Read the model definition and answer for the solid it produces. Units are mm, in the model's axes. A direction names the side the tool comes from. Give positions to 0.01 mm unless a question says otherwise; leave off trailing zeros. Write each loop counter-clockwise with the first axis right and the second up, starting at its lowest first coordinate (ties: lowest second). Pieces come first, ordered by that corner, then holes. Notation, with made-up numbers: M 86.25,74 L 90.25,74 A22 cw 90.25,110 Z; hole C 40,-22 d10. An arc over 180 degrees is marked long. Answer as CSV lines item,"result". Start each with the question number.
```python
from build123d import *

# Parameters (mm, degrees)
SKETCH2_W          = 20.32
SKETCH2_H          = 20.32
CENTRAL_BOX_DEPTH  = 25.4
NIBBLES_DEPTH      = 6.35
NIBBLES_DEPTH_BACK = 31.75
SKETCH4_R          = 3.175
YAY_ROUNDED_R      = 2.54


with BuildPart() as part:
    # Sketch2 → central box (new body)
    with BuildSketch(Plane(origin=(0, 0, 0), x_dir=(0, 0, -1), z_dir=(1, 0, 0))):
        with Locations((10.16, 10.16)):
            Rectangle(SKETCH2_W, SKETCH2_H)
    extrude(amount=CENTRAL_BOX_DEPTH)

    # Sketch4 → nibbles (add, two sides: drawn at the far end of the back side and taken through both)
    with BuildSketch(Plane(origin=(25.4, 0, 0), x_dir=(0, 0, -1), z_dir=(1, 0, 0)).offset(-NIBBLES_DEPTH_BACK)):
        with Locations((10.16, 10.16)):
            Circle(SKETCH4_R)
    extrude(amount=NIBBLES_DEPTH + NIBBLES_DEPTH_BACK)

    # Sketch6 → stick (revolve)
    with BuildSketch(Plane.XY.offset(-10.16), mode=Mode.PRIVATE) as stick_sk:
        with BuildLine():
            Line((12.7, 20.32), (12.7, 48.26))
            Line((12.7, 48.26), (22.69993783, 48.26))
            Line((22.69993783, 48.26), (22.69993783, 43.18))
            add(Edge.make_bspline(
                [(22.69993783, 43.18), (14.011650276, 53.987913913), (15.389137078, 36.935795993), (15.494, 20.32)],
                knots=[0, 0, 0, 0, 1, 1, 1, 1], degree=3))
            Line((15.494, 20.32), (12.7, 20.32))
        make_face()
    revolve(stick_sk.sketch.rotate(Axis((12.7, 20.32, -10.16), (0, 1, 0)), 90), axis=Axis((12.7, 20.32, -10.16), (0, 1, 0)))

    # yay, rounded
    yay_rounded_edges = [part.edges().sort_by_distance(p)[0] for p in [
        (12.7, 20.32, -7.366),
        (12.7, 48.26, -0.16006217),
    ]]
    fillet(yay_rounded_edges, radius=YAY_ROUNDED_R)


solid = part.part
```
1. Find section A-A on y = 10.16. Determine the outline of the cut face in (x, z) (3 decimals), then the cut area to 3 significant figures.
2. Find section B-B on x = -1. Determine the outline of the cut face in (y, z) (3 decimals).
3. For faces 4 (the face through (13, 0, -10)), 5 (the face through (25.4, 13, -8)), 6 (the face through (-3.22, 11.11, -13.19)), determine the directions among +Z, -Z, +X, -X, +Y, -Y from which every point of the face is accessible in a straight line to the end or side of a thin tool.
4. Find the intervals of material crossed by line 1 (Y direction, x = 17, z = -14); line 2 (X direction, y = 4, z = -18.5); line 3 (Y direction, x = 8, z = -11), in increasing order. Write a range as [from, to].
5. Find section C-C on y = 18.5. Determine the outline of the cut face in (x, z).
6. Given pin 1 (10 mm diameter, centred on x = 23, z = -11.5, fed in from -Y); pin 2 (1.5 mm diameter, centred on x = 13.5, y = 27.5, fed in from +Z); pin 3 (4 mm diameter, centred on x = 20.5, z = -16.5, fed in from +Y); pin 4 (4 mm diameter, centred on x = 25.5, z = -7.5, fed in from +Y), each flat-ended and moving along its own axis, determine where each tip first touches the part or whether it passes through.
7. Determine the mould class of faces 1 (the face through (2.785, 44.432, -8.858)), 2 (the face through (13, 48.26, -10)), 3 (the face through (9.7, 20.32, -5.5)) for opening direction Y: +Y half, -Y half, draft (parallel to the pull), parting line (faces both ways), or undercut.
Computed:
1,outline,"M -6.35,-13.335 L 0,-13.335 L 0,-20.32 L 25.4,-20.32 L 25.4,-13.335 L 31.75,-13.335 L 31.75,-6.985 L 25.4,-6.985 L 25.4,0 L 0,0 L 0,-6.985 L -6.35,-6.985 Z"
1,area,"597 mm^2"
2,outline,"C 10.16,-10.16 d6.35"
3,face 4,"+Z, -Z, +X, -X, -Y"
3,face 5,"+X"
3,face 6,"-X"
4,line 1,"y = [0, 20.32], [46.56, 48.26]"
4,line 2,"x = [0, 25.4]"
4,line 3,"y = [0, 20.38], [46.3, 48.26]"
5,outline,"M 0,-20.32 L 25.4,-20.32 L 25.4,0 L 0,0 Z"
6,pin 1,"stops at y = 0"
6,pin 2,"stops at z = -7.46"
6,pin 3,"stops at y = 48.19"
6,pin 4,"stops at y = 20.32"
7,face 1,"draft"
7,face 2,"+Y half"
7,face 3,"undercut"
